from build123d import *

# Parameters (mm, degrees)
F0_R     = 2
F1_DEPTH = 1.5
F2_R     = 4
F3_R     = 10
F4_R     = 4


with BuildPart() as f1:
    # F0 (on Top) → F1 (new body)
    with BuildSketch(Plane.XY):
        Polygon((6, 3.5), (3, 10.5), (-3, 10.5), (-6, 3.5), (-6, -10.5), (6, -10.5), align=None)
        with BuildLine():
            ThreePointArc((-2, -8.5), (-4, -6.5), (-2, -4.5))
            Line((-2, -4.5), (2, -4.5))
            ThreePointArc((2, -4.5), (3.414214, -5.085786), (4, -6.5))
            ThreePointArc((4, -6.5), (3.414214, -7.914214), (2, -8.5))
            Line((2, -8.5), (-2, -8.5))
        make_face(mode=Mode.SUBTRACT)
        with BuildLine():
            ThreePointArc((-2, -2.5), (-4, -0.5), (-2, 1.5))
            Line((-2, 1.5), (2, 1.5))
            ThreePointArc((2, 1.5), (3.414214, 0.914214), (4, -0.5))
            ThreePointArc((4, -0.5), (3.414214, -1.914214), (2, -2.5))
            Line((2, -2.5), (-2, -2.5))
        make_face(mode=Mode.SUBTRACT)
        with Locations((0, 6.5)):
            Circle(F0_R, mode=Mode.SUBTRACT)
    extrude(amount=F1_DEPTH)

    # F2
    f2_edges = [f1.edges().sort_by_distance(p)[0] for p in [
        (3, 10.5, 0.75),
        (-3, 10.5, 0.75),
    ]]
    fillet(f2_edges, radius=F2_R)

    # F3
    f3_edges = [f1.edges().sort_by_distance(p)[0] for p in [
        (-6, 3.5, 0.75),
        (6, 3.5, 0.75),
    ]]
    fillet(f3_edges, radius=F3_R)

    # F4
    f4_edges = [f1.edges().sort_by_distance(p)[0] for p in [
        (-6, -10.5, 0.75),
        (6, -10.5, 0.75),
    ]]
    fillet(f4_edges, radius=F4_R)


solid = f1.part
Geometry: final body of the model. Coordinates: model frame, mm. A direction names the side the tool comes from. Give positions to 0.01 mm unless a question says otherwise; leave off trailing zeros. Order: outer loops, then holes, each group sorted by start corner. A loop starts at its lowest first (then second) coordinate and runs counter-clockwise, first axis right, second up. Notation, with made-up numbers: (84, 36.25) -> (141, 36.25) arc R7 cw to (141, 49.25) -> close; hole circle Ø9 at (2, 12). An arc over 180 degrees is marked (long way). Answer as a JSON object with one key per item and string values.
Q1. Material intervals for probe 1 along Y at (x, z) = (0, 1.1); probe 2 along Y at (x, z) = (-0.5, 0.75); probe 3 along Y at (x, z) = (3.5, 0.9), sorted ascending.
Entries:
{"probe 1": "y = -10.5 to -8.5, -4.5 to -2.5, 1.5 to 4.5, 8.5 to 10.5", "probe 2": "y = -10.5 to -8.5, -4.5 to -2.5, 1.5 to 4.56, 8.44 to 10.5", "probe 3": "y = -10.21 to -7.82, -5.18 to -1.82, 0.82 to 8.98"}
Q2. First-contact query: pin 1 (2.5 mm diameter, centred on x = 0, y = 6.5, fed in from -Z). Flat tip, straight axial feed; report the tip coordinate or a pass-through.
Entries:
{"pin 1": "passes through"}
Q3. Section D-D (x = -3.75). Output: boundary loops of the cut face in (y, z), plus the area to 3 significant figures.
Entries:
{"outline": "(-10.1, 0) -> (-7.47, 0) -> (-7.47, 1.5) -> (-10.1, 1.5) -> close; (-5.53, 0) -> (-1.47, 0) -> (-1.47, 1.5) -> (-5.53, 1.5) -> close; (0.47, 0) -> (8.63, 0) -> (8.63, 1.5) -> (0.47, 1.5) -> close", "area": "22.3 mm^2"}
Q4. Draft query along Y for faces 3 (the cylindrical face through (-4.797, -9.359, 0.76)), 4 (the flat face through (4.623, 6.712, 0.74)), 5 (the cylindrical face through (-4, -0.5, 0.7)). Return one class per face: released by +Y, released by -Y, zero draft, split by the parting line, or undercut.
Entries:
{"face 3": "released by -Y", "face 4": "released by +Y", "face 5": "undercut"}
Q5. Section C-C (y = 6.5). Output: boundary loops of the cut face in (x, z).
Entries:
{"outline": "(-4.71, 0) -> (-2, 0) -> (-2, 1.5) -> (-4.71, 1.5) -> close; (2, 0) -> (4.71, 0) -> (4.71, 1.5) -> (2, 1.5) -> close"}
Q6. Access query for faces 1 (the cylindrical face through (2.59, 9.82, 0.76)), 2 (the flat face through (0, -2.5, 1)). Directions: +Z, -Z, +X, -X, +Y, -Y. A direction counts if a zero-diameter tool reaches every point of the face in a straight line with its end or side. Return the directions, or none.
Entries:
{"face 1": "+Z, -Z, +X, +Y", "face 2": "+Z, -Z"}
Q7. Section A-A (z = 0.6). Output: boundary loops of the cut face in (x, y).
Entries:
{"outline": "(-6, -6.5) arc R4 ccw to (-2, -10.5) -> (2, -10.5) arc R4 ccw to (6, -6.5) -> (6, 1.45) arc R10 ccw to (5.19, 5.39) -> (4.04, 8.08) arc R4 ccw to (0.36, 10.5) -> (-0.36, 10.5) arc R4 ccw to (-4.04, 8.08) -> (-5.19, 5.39) arc R10 ccw to (-6, 1.45) -> close; hole (-2, -8.5) -> (2, -8.5) arc R2 ccw to (4, -6.5) arc R2 ccw to (2, -4.5) -> (-2, -4.5) arc R2 ccw to start; hole (-2, -2.5) -> (2, -2.5) arc R2 ccw to (4, -0.5) arc R2 ccw to (2, 1.5) -> (-2, 1.5) arc R2 ccw to start; hole circle Ø4 at (0, 6.5)"}
Q8. Section B-B (x = 0). Output: boundary loops of the cut face in (y, z), plus the area to 3 significant figures.
Entries:
{"outline": "(-10.5, 0) -> (-8.5, 0) -> (-8.5, 1.5) -> (-10.5, 1.5) -> close; (-4.5, 0) -> (-2.5, 0) -> (-2.5, 1.5) -> (-4.5, 1.5) -> close; (1.5, 0) -> (4.5, 0) -> (4.5, 1.5) -> (1.5, 1.5) -> close; (8.5, 0) -> (10.5, 0) -> (10.5, 1.5) -> (8.5, 1.5) -> close", "area": "13.5 mm^2"}
